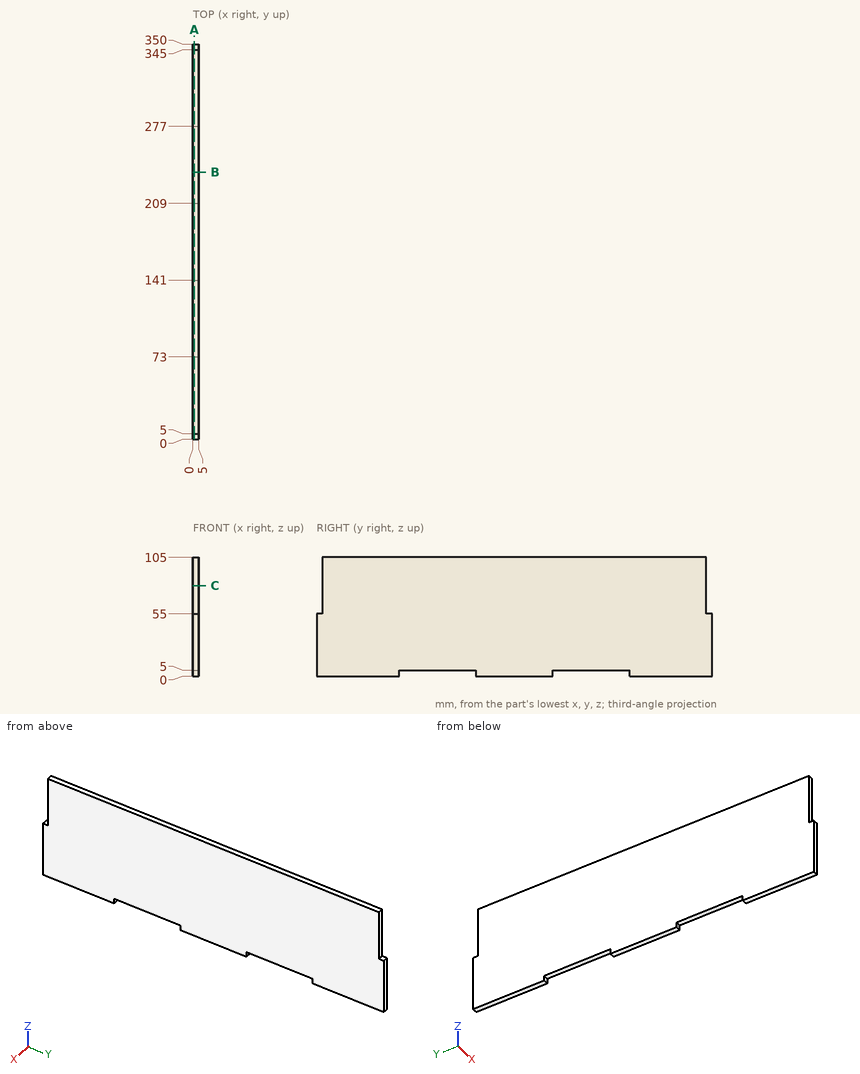
Check sheet for the drawn part. Datum: minimum x, y, z corner. Units: mm. Give positions to 0.01 mm unless a question says otherwise; leave off trailing zeros. Write each loop counter-clockwise with the first axis right and the second up, starting at its lowest first coordinate (ties: lowest second). Pieces come first, ordered by that corner, then holes. Notation, with made-up numbers: M 12.25,81.25 L 36.25,81.25 A15 cw 36.25,93.25 Z; hole C 57,73.5 d6. An arc over 180 degrees is marked long. One line per question, with ' | ' between items.
1. Cross-section at A-A (x = 1.3). Enter the section's corners in (y, z), plus the area to 3 significant figures.
Ans:
outline: M 0,0 L 73,0 L 73,5 L 141,5 L 141,0 L 209,0 L 209,5 L 277,5 L 277,0 L 350,0 L 350,55 L 345,55 L 345,105 L 5,105 L 5,55 L 0,55 Z | area: 35,600 mm2
2. Cross-section at B-B (y = 236.5). Enter the section's corners in (x, z).
Ans:
outline: M 0,5 L 5,5 L 5,105 L 0,105 Z
3. Gauge pin test, flat ends, axial feed: pin 1 (1.5 mm diameter, centred on x = 2.5, y = 103, fed in from -Z); pin 2 (2.5 mm diameter, centred on x = 1.5, y = 347, fed in from +Z); pin 3 (2.5 mm diameter, centred on x = 2, z = 89, fed in from +Y). Record the tip position at first contact, or that the pin passes through.
Ans:
pin 1: z = 5 | pin 2: z = 55 | pin 3: y = 345
4. Scan lines: line 1 along Y through (x, z) = (4.7, 69.5); line 2 along Z through (x, y) = (1.3, 217). Record each from-to range of solid material in increasing order. Write a range as from..to.
Ans:
line 1: 5..345 | line 2: 5..105
5. Cross-section at C-C (z = 80). Enter the section's corners in (x, y).
Ans:
outline: M 0,5 L 5,5 L 5,345 L 0,345 Z
